CAD build for the part. Positions are in the model's coordinates, mm. A direction names the side the tool comes from. Give positions to 0.01 mm unless a question says otherwise; leave off trailing zeros. Order: outer loops, then holes, each group sorted by start corner. A loop starts at its lowest first (then second) coordinate and runs counter-clockwise, first axis right, second up.
```python
from build123d import *

# Parameters (mm, degrees)
CROQUIS1_W              = 15
CROQUIS1_H              = 50
CROQUIS1_W_2            = 50
CROQUIS1_H_2            = 115
SALIENTE_EXTRUIR1_DEPTH = 250
CROQUIS2_R              = 80
SALIENTE_EXTRUIR2_DEPTH = 35


with BuildPart() as part:
    # Croquis1 → Saliente-Extruir1 (new body)
    with BuildSketch(Plane(origin=(0, 0, 0), x_dir=(1, 0, 0), z_dir=(0, 1, 0))):
        with Locations((-32.5, 0)):
            Rectangle(CROQUIS1_W, CROQUIS1_H)
        Rectangle(CROQUIS1_W_2, CROQUIS1_H_2)
    extrude(amount=SALIENTE_EXTRUIR1_DEPTH)

    # Croquis2 → Saliente-Extruir2 (add)
    with BuildSketch(Plane(origin=(0, 250, 0), x_dir=(1, 0, 0), z_dir=(0, 1, 0))):
        with Locations(Location((-25, 0, 0), (0, 0, 270))):
            Circle(CROQUIS2_R)
    extrude(amount=SALIENTE_EXTRUIR2_DEPTH)


solid = part.part
```
Item 1: Wall check: L1, parallel to Y at x = -66, z = 49.5; L2, parallel to X at y = 214.5, z = 8; L3, parallel to X at y = 109.5, z = 35. Give the ranges that are in metal, low to high.
Item 2: Slice it at B-B (z = 0). Give the cut face in (x, y).
Item 3: Drop flat-ended pins along their axis: pin 1 Ø25 at (x, y) = (2.5, 100.5) entering from +Z; pin 2 Ø5 at (y, z) = (216.5, 0) entering from +X; pin 3 Ø7.5 at (x, y) = (-29.5, 79) entering from +Z. Give the stop position or say it passes through.
Item 4: Slice it at C-C (y = 259.5). Give the cut face in (x, z).
Item 5: Tool access for faces 1 (the face through (-40, 123, 0)), 2 (the face through (-33, 123, 25)), 3 (the face through (25, 123, 1)): list every direction of +Z, -Z, +X, -X, +Y, -Y with a clear straight run to the whole face (end or side of a thin tool).
Item 6: Slice it at A-A (y = 112). Give the cut face in (x, z), and give its area (3 significant figures).
A:
1. L1: y = 250 to 285
1. L2: x = -40 to 25
1. L3: x = -25 to 25
2. outline: (-105, 250) - (-40, 250) - (-40, 0) - (25, 0) - (25, 250) - (55, 250) - (55, 285) - (-105, 285) - close
3. pin 1: stops at z = 57.5
3. pin 2: stops at x = 25
3. pin 3: stops at z = 25
4. outline: circle Ø160 at (-25, 0)
5. face 1: +Z, -Z, -X, -Y
5. face 2: +Z, -X, -Y
5. face 3: +Z, -Z, +X, -Y
6. outline: (-40, -25) - (-25, -25) - (-25, -57.5) - (25, -57.5) - (25, 57.5) - (-25, 57.5) - (-25, 25) - (-40, 25) - close
6. area: 6,500 mm2
